Can you work these out from the drawing? Everything is in mm from the part's minimum corner. Give positions to 0.01 mm unless a question says otherwise; leave off trailing zeros. Order: outer loops, then holes, each group sorted by start corner. A loop starts at its lowest first (then second) coordinate and runs counter-clockwise, first axis right, second up. Notation, with made-up numbers: (7.5, 42) - (58.5, 42) arc R22 cw to (58.5, 48) - close; hole circle Ø1 at (22.25, 86). An arc over 180 degrees is marked (long way). One line per question, with ' | ' between items.
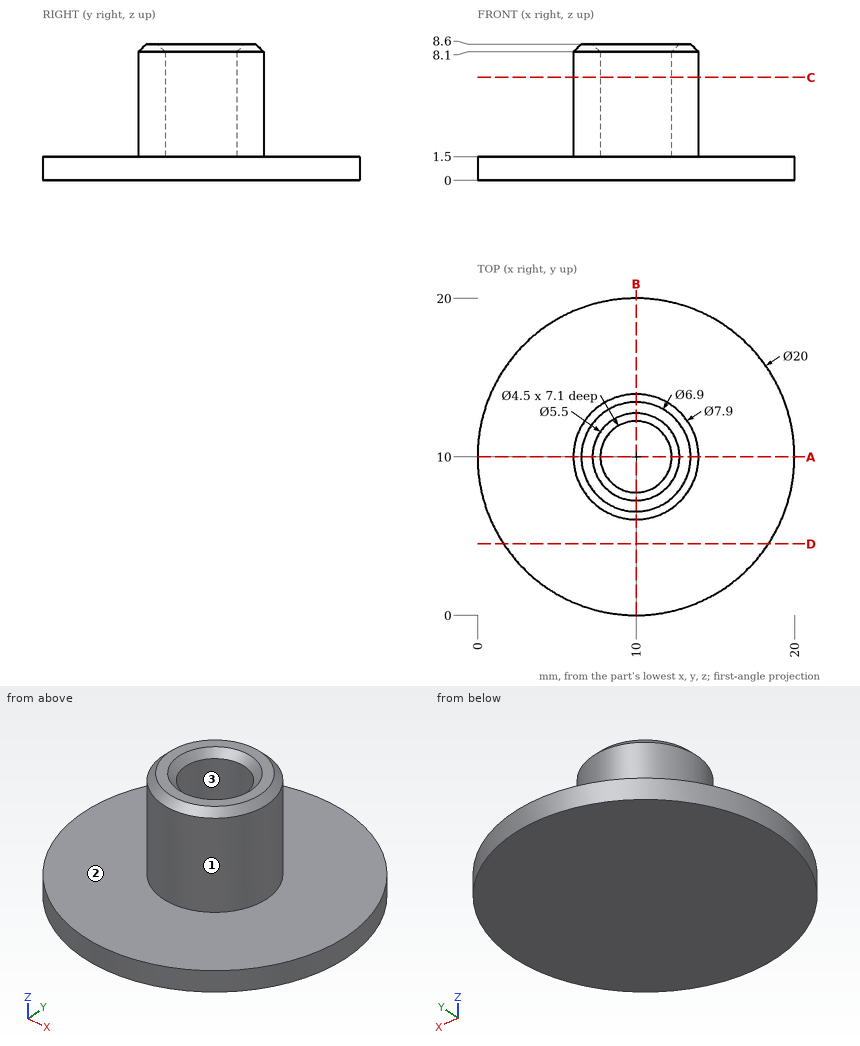
(1) Will these pins go through, and if not, where does the flat tip stop? pin 1 (3 mm diameter, centred on x = 8, y = 15.5, fed in from +Z); pin 2 (5 mm diameter, centred on x = 6.5, z = 3.5, fed in from -Y); pin 3 (2 mm diameter, centred on y = 14, z = 4, fed in from +X).
Answer below:
pin 1: z = 1.5 | pin 2: y = 0.2 | pin 3: x = 12.57
(2) If we mould it in two halves opening along Y, with no side actions, what happens to the marked faces 1, 2 and 3? For each: released by +Y, released by -Y, zero draft, split by the parting line, or undercut.
Answer below:
face 1: split by the parting line | face 2: zero draft | face 3: undercut
(3) If I drill on line 1 (Y direction, x = 10, z = 3.75); line 2 (Z direction, x = 16, y = 17.5); line 3 (X direction, y = 8, z = 5.5), over which ranges is the centre line in solid material (lowest first)?
Answer below:
line 1: 6.05 to 7.75, 12.25 to 13.95 | line 2: 0 to 1.5 | line 3: 6.59 to 8.97, 11.03 to 13.41
(4) Imagine slicing it at A-A (y = 10). List the corners of the cut face in (x, z) for me, and give its area (3 significant figures).
Answer below:
outline: (0, 0) - (20, 0) - (20, 1.5) - (13.95, 1.5) - (13.95, 8.1) - (13.45, 8.6) - (12.75, 8.6) - (12.25, 8.1) - (12.25, 1.5) - (7.75, 1.5) - (7.75, 8.1) - (7.25, 8.6) - (6.55, 8.6) - (6.05, 8.1) - (6.05, 1.5) - (0, 1.5) - close | area: 53.6 mm^2
(5) Imagine slicing it at C-C (z = 6.5). List the corners of the cut face in (x, y) for me.
Answer below:
outline: circle Ø7.9 at (10, 10); hole circle Ø4.5 at (10, 10)
(6) Imagine slicing it at D-D (y = 4.5). List the corners of the cut face in (x, z) for me, and give its area (3 significant figures).
Answer below:
outline: (1.65, 0) - (18.35, 0) - (18.35, 1.5) - (1.65, 1.5) - close | area: 25.1 mm^2
